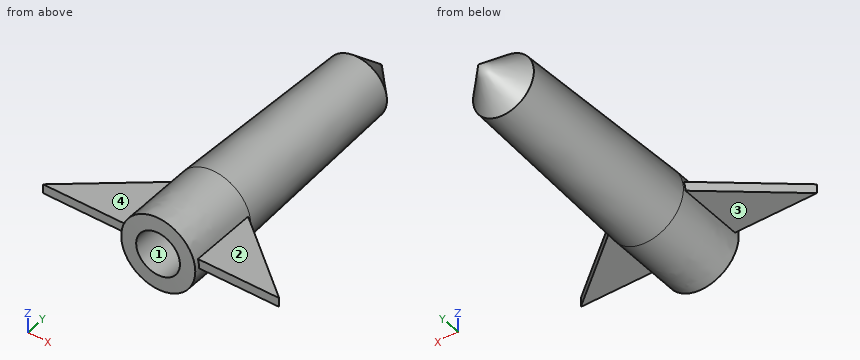
```python
from build123d import *

# Parameters (mm, degrees)
F3_DEPTH = 4.572
F4_R     = 10.922
F5_DEPTH = 88.392


with BuildPart() as f1:
    # F0 (on Top) → F1 (revolve)
    with BuildSketch(Plane.XY):
        Polygon((-19.2241743207, 52.9774539173), (-34.4217829406, 69.6123968682), (-34.360922873, -78.7533447146), (-15.8556289971, -78.3891752362), (-15.8556289971, -41.6480451822), align=None)
    revolve(axis=Axis((-34.3913529068, -4.5704739232, 0), (0.0004102029, -0.9999999159, 0)))

    # F2 (on Top) → F3 (join)
    with BuildSketch(Plane.XY):
        Polygon((-52.7703391896, -75.8608434159), (-52.4374330146, -42.6783543754), (-93.8421391896, -75.8608434159), align=None)
        Polygon((24.1632689069, -75.8608434159), (-16.9141878514, -42.2792753768), (-16.9141878514, -75.8608434159), align=None)
    extrude(amount=F3_DEPTH)

    # F4 (on Front) → F5 (cut)
    with BuildSketch(Plane.XZ):
        with Locations((-34.3477502465, 0)):
            Circle(F4_R)
    extrude(amount=F5_DEPTH, mode=Mode.SUBTRACT)


solid = f1.part
```
The model under review builds one solid part; all positions refer to its coordinate system, in mm. Face numbers are marked on the shaded views. A direction names the side the tool comes from. Round coordinates to 2 decimals unless told otherwise and drop trailing zeros. Order: outer loops, then holes, each group sorted by start corner. A loop starts at its lowest first (then second) coordinate and runs counter-clockwise, first axis right, second up.
(1) For P1, Ø5, axis at x = 10, z = 2.5, coming from the -Y side; P2, Ø4, axis at x = -22, y = -15, coming from the +Z side; P3, Ø11, axis at x = -30.5, z = -5, coming from the -Y side, all flat-tipped, find the tip position at first contact; note any pin that passes through.
Working result:
P1: stops at y = -75.86
P2: stops at z = 14.19
P3: stops at y = -78.54
(2) Tool access review of the marked faces 1, 2, 3 and 4: name each direction out of +Z, -Z, +X, -X, +Y, -Y from which nothing blocks a thin tool from reaching the whole face with its end or side.
Working result:
face 1: -Y
face 2: +Z, +X, +Y, -Y
face 3: -Z, -X, +Y, -Y
face 4: +Z, -X, +Y, -Y
(3) Wall thickness on L1, parallel to Z at x = 3, y = -68; L2, parallel to X at y = -0.5, z = -4; L3, parallel to X at y = -15, z = -1: over which ranges is each line inside the solid? List them lowest first.
Working result:
L1: z = 0 to 4.57
L2: x = -50.99 to -44.51, -24.18 to -17.8
L3: x = -51.94 to -45.22, -23.47 to -16.83
(4) Take a section at A-A, the plane x = -56.5. State the section outline as (y, z) points.
Working result:
outline: (-75.86, 0) - (-45.93, 0) - (-45.93, 4.57) - (-75.86, 4.57) - close
